Autodesk Inventor part; units mm, degrees
ref_plane "YZ Plane" through (0, 0, 0) normal (1, 0, 0) x (0, 1, 0)
ref_plane "XZ Plane" through (0, 0, 0) normal (0, 1, 0) x (-1, 0, 0)
ref_plane "XY Plane" through (0, 0, 0) normal (0, 0, 1) x (1, 0, 0)
sketch "Sketch1" plane through (0, 0, 0) normal (0, 0, 1) x (1, 0, 0)
  line L0 (0, 0) -> (0, 1.6)
  line L1 (0, 1.6) -> (-24, 1.6)
  line L2 (-24, 1.6) -> (-24, 0)
  line L3 (-24, 0) -> (0, 0)
  line L4 (0, 1.6) -> (8, 17.6)
  line L5 (8, 17.6) -> (-8, 17.6)
  line L6 (-8, 17.6) -> (-24, 1.6)
  line L7 (-8, 17.6) -> (-8, 19.2)
  line L8 (-8, 19.2) -> (8, 19.2)
  line L9 (8, 19.2) -> (8, 17.6)
  dimension "d0" = 16
  dimension "d1" = 24
  dimension "d2" = 1.6
  dimension "d3" = 1.6
  dimension "d4" = 19.2
  dimension "d5" = 8
extrude "Extrusion1" add sketch "Sketch1" along normal mid plane 16 contours L5 L7 L8 L9
extrude "Extrusion2" add sketch "Sketch1" along normal mid plane 8 contours L3 L2 L1 L0
extrude "Extrusion3" add sketch "Sketch1" along normal mid plane 1.6 contours L1 L6 L5 L4
sketch "Sketch2" plane through (-8, 19.2, 8) normal (0, 1, 0) x (1, 0, 0)
  line L0 (16, 16) -> (0, 16)
  line L1 (0, 16) -> (0, 0)
  circle A0 centre (4, 12) radius 2.5
  circle A1 centre (4, 12) radius 1.5
  circle A2 centre (12, 12) radius 1.5
  circle A3 centre (12, 12) radius 2.5
  circle A4 centre (4, 4) radius 1.5
  circle A5 centre (4, 4) radius 2.5
  circle A6 centre (12, 4) radius 1.5
  circle A7 centre (12, 4) radius 2.5
  point P0 (8, 8)
  dimension "d12" = 5
  dimension "d13" = 4
  dimension "d14" = 8
  dimension "d15" = 4
  dimension "d16" = 8
  dimension "d17" = 3
extrude "Extrusion4" add sketch "Sketch2" along normal blind 1.6
sketch "Sketch3" plane through (-24, 0, 4) normal (0, -1, 0) x (1, 0, 0)
  line L0 (24, 0) -> (0, 0)
  line L1 (0, -8) -> (0, 0)
  line L2 (0, -8) -> (24, -8)
  line L3 (24, 0) -> (24, -8)
  line L4 (22.8868, 0) -> (21.4434, -2.5)
  line L5 (21.4434, -2.5) -> (18.5566, -2.5)
  line L6 (18.5566, -2.5) -> (17.1132, 0)
  circle A0 centre (20, 0) radius 2.5 construction
  line L7 (14.8868, 0) -> (13.4434, -2.5)
  line L8 (13.4434, -2.5) -> (10.5566, -2.5)
  line L9 (10.5566, -2.5) -> (9.1132, 0)
  circle A1 centre (12, 0) radius 2.5 construction
  line L10 (6.8868, 0) -> (5.4434, -2.5)
  line L11 (5.4434, -2.5) -> (2.5566, -2.5)
  line L12 (2.5566, -2.5) -> (1.1132, 0)
  circle A2 centre (4, 0) radius 2.5 construction
  line L13 (0, -4) -> (24, -4) construction
  line L14 (0, -4) -> (24, -4)
  line L15 (22.8868, -8) -> (21.4434, -5.5)
  line L16 (21.4434, -5.5) -> (18.5566, -5.5)
  line L17 (18.5566, -5.5) -> (17.1132, -8)
  line L18 (10.5566, -5.5) -> (9.1132, -8)
  line L19 (13.4434, -5.5) -> (10.5566, -5.5)
  line L20 (14.8868, -8) -> (13.4434, -5.5)
  line L21 (2.5566, -5.5) -> (1.1132, -8)
  line L22 (5.4434, -5.5) -> (2.5566, -5.5)
  line L23 (6.8868, -8) -> (5.4434, -5.5)
  line L24 (2.5566, -5.5) -> (0, -5.5)
  line L25 (2.5566, -2.5) -> (0, -2.5)
  line L26 (1.1132, -8) -> (6.8868, -8)
  line L27 (9.1132, -8) -> (14.8868, -8)
  line L28 (17.1132, -8) -> (22.8868, -8)
  line L29 (22.8868, 0) -> (17.1132, 0)
  line L30 (14.8868, 0) -> (9.1132, 0)
  line L31 (6.8868, 0) -> (1.1132, 0)
  line L32 (1.1132, 0) -> (0, 0)
  line L33 (0, 0) -> (0, -2.5)
  line L34 (0, -5.5) -> (0, -8)
  line L35 (0, -8) -> (1.1132, -8)
  point P0 (20, -8)
  point P1 (12, -8)
  point P2 (4, -8)
  dimension "d20" = 5
  dimension "d21" = 4
  dimension "d22" = 120
  dimension "d25" = 8
extrude "Extrusion5" cut sketch "Sketch3" against normal blind 1.6 contours L4 L5 L6 L0 | L7 L8 L9 L0 | L2 L17 L16 L15 | L24 L21 L2 L1 | L1 L0 L12 L25 | L22 L23 L2 L21 | L12 L0 L10 L11 | L2 L18 L19 L20
properties part number "3479" material "Steel"
Could you check a few things on this model? Use its own coordinates, in mm. A direction names the side the tool comes from. Round coordinates to 2 decimals unless told otherwise and drop trailing zeros. Loops run counter-clockwise (first coordinate to the right, second up) from the corner with the lowest first, then second, coordinate; pieces in that order, holes last. Notation, with made-up numbers: (-40, 0.5) -> (4, 0.5) arc R20 ccw to (4, 26.5) -> close; hole circle Ø8 at (56, 48). An arc over 180 degrees is marked (long way). Use CSV: the item, a comma, the result in double quotes.
(1) Suppose I cut it at A-A on x = -4. Write out the boundary of the cut face in (y, z), plus the area to 3 significant figures.
Return value:
outline,"(0, -1.5) -> (1.6, -1.5) -> (1.6, -0.8) -> (17.6, -0.8) -> (17.6, -8) -> (19.2, -8) -> (19.2, -6.5) -> (20.8, -6.5) -> (20.8, -5.5) -> (19.2, -5.5) -> (19.2, -2.5) -> (20.8, -2.5) -> (20.8, -1.5) -> (19.2, -1.5) -> (19.2, 1.5) -> (20.8, 1.5) -> (20.8, 2.5) -> (19.2, 2.5) -> (19.2, 5.5) -> (20.8, 5.5) -> (20.8, 6.5) -> (19.2, 6.5) -> (19.2, 8) -> (17.6, 8) -> (17.6, 0.8) -> (1.6, 0.8) -> (1.6, 1.5) -> (0, 1.5) -> close"
area,"62.4 mm²"
(2) If I drill on probe 1 along X at (y, z) = (20, 4); probe 2 along X at (y, z) = (19.5, -3), over which ranges is the centre line in solid material (lowest first)? Write a range as [from, to].
Return value:
probe 1,"x = [-6.5, -5.5], [-2.5, -1.5], [1.5, 2.5], [5.5, 6.5]"
probe 2,"x = [-6.29, -5.12], [-2.88, -1.71], [1.71, 2.88], [5.12, 6.29]"
(3) Suppose I cut it at B-B on z = -0.25. Write out the boundary of the cut face in (x, y).
Return value:
outline,"(-24, 0) -> (0, 0) -> (0, 1.6) -> (8, 17.6) -> (8, 19.2) -> (-8, 19.2) -> (-8, 17.6) -> (-24, 1.6) -> close"
(4) Suppose I cut it at C-C on y = 15. Write out the boundary of the cut face in (x, z), plus the area to 3 significant figures.
Return value:
outline,"(-10.6, -0.8) -> (6.7, -0.8) -> (6.7, 0.8) -> (-10.6, 0.8) -> close"
area,"27.7 mm²"
(5) Will these pins go through, and if not, where does the flat tip stop? pin 1 Ø1.3 at (y, z) = (18.5, -2) entering from -X; pin 2 Ø0.8 at (x, y) = (-22, 0.5) entering from -Z; pin 3 Ø1.8 at (x, y) = (-16, 0.5) entering from -Z; pin 4 Ø1.5 at (x, y) = (-13.5, 13.5) entering from +Z.
Return value:
pin 1,"stops at x = -8"
pin 2,"stops at z = -1.5"
pin 3,"stops at z = -4"
pin 4,"passes through"
(6) Suppose I cut it at D-D on x = -16. Write out the boundary of the cut face in (y, z).
Return value:
outline,"(0, -4) -> (1.6, -4) -> (1.6, -0.8) -> (9.6, -0.8) -> (9.6, 0.8) -> (1.6, 0.8) -> (1.6, 4) -> (0, 4) -> close"
(7) For faces 5 (the flat face through (-14.155, 0.789, -2.733)), 6 (the flat face through (-0.6, 0.8, -4)), 7 (the flat face through (-21, 1, -1.5)), 8 (the flat face through (-9.825, 0.789, 2.767)), which set-ups out of +Z, -Z, +X, -X, +Y, -Y let a thin tool reach every point of the face, with its end or its side?
Return value:
face 5,"-Z, +Y, -Y"
face 6,"-Z, +X, -X, -Y"
face 7,"-Z, -X, +Y, -Y"
face 8,"+Z, +Y, -Y"
(8) If we mould it in two halves opening along Z, with no side actions, what happens to faces 1 (the flat face through (-4, 19.2, -4)), 2 (the flat face through (-15.9, 9.7, 0)), 3 (the flat face through (-6.155, 0.789, 2.733)), 4 (the flat face through (-4, 1, -1.5))? For each: +Z half, -Z half, draft (parallel to the pull), parting line (faces both ways), or undercut.
Return value:
face 1,"undercut"
face 2,"draft"
face 3,"+Z half"
face 4,"-Z half"
